Could you check a few things on this model? Use its own coordinates, in mm. Face numbers are marked on the shaded views. A direction names the side the tool comes from. Coordinates: 2 decimals unless noted, no trailing zeros. Loops run counter-clockwise (first coordinate to the right, second up) from the corner with the lowest first, then second, coordinate; pieces in that order, holes last.
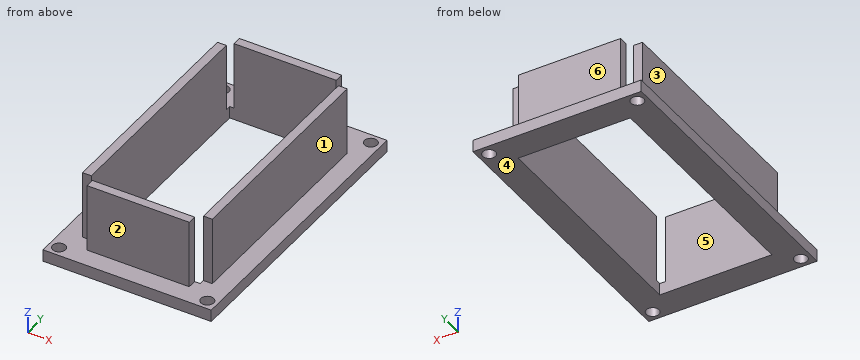
from build123d import *

# Parameters (mm, degrees)
F0_W     = 42
F0_H     = 72
F0_R     = 1.6
F1_DEPTH = 3
F0_W_2   = 25.488504
F0_H_2   = 2.2
F0_W_3   = 2.2
F0_H_3   = 55.283766
F2_DEPTH = 20


with BuildPart() as f1:
    # F0 (on Top) → F1 (new body)
    with BuildSketch(Plane.XY):
        with Locations((-2.088945, 1.718141)):
            Rectangle(F0_W, F0_H)
        with Locations((-20.588945, -31.781859)):
            Circle(F0_R, mode=Mode.SUBTRACT)
        with Locations((16.411055, -31.781859)):
            Circle(F0_R, mode=Mode.SUBTRACT)
        with Locations((-20.588945, 35.218141)):
            Circle(F0_R, mode=Mode.SUBTRACT)
        Polygon((-18.288945, 32.918141), (-14.99591, 32.918141), (10.492594, 32.918141), (14.111055, 32.918141), (14.111055, 29.307075), (14.111055, -25.976691), (14.111055, -27.281859), (14.111055, -29.481859), (10.492594, -29.481859), (-14.99591, -29.481859), (-18.288945, -29.481859), (-18.288945, -25.976691), (-18.288945, 29.307075), align=None, mode=Mode.SUBTRACT)
        with Locations((16.411055, 35.218141)):
            Circle(F0_R, mode=Mode.SUBTRACT)
        Polygon((-16.088945, -27.281859), (-16.088945, -25.976691), (-18.288945, -25.976691), (-18.288945, -29.481859), (-14.99591, -29.481859), (-14.99591, -27.281859), align=None)
        Polygon((-16.088945, 29.307075), (-16.088945, 30.718141), (-14.99591, 30.718141), (-14.99591, 32.918141), (-18.288945, 32.918141), (-18.288945, 29.307075), align=None)
        Polygon((10.492594, 32.918141), (10.492594, 30.718141), (11.911055, 30.718141), (11.911055, 29.307075), (14.111055, 29.307075), (14.111055, 32.918141), align=None)
        Polygon((14.111055, -25.976691), (11.911055, -25.976691), (11.911055, -27.281859), (10.492594, -27.281859), (10.492594, -29.481859), (14.111055, -29.481859), (14.111055, -27.281859), align=None)
    extrude(amount=F1_DEPTH)

    # F0 (on Top) → F2 (join)
    with BuildSketch(Plane.XY):
        with Locations((-2.251658, 31.818141)):
            Rectangle(F0_W_2, F0_H_2)
        with Locations((-17.188945, 1.665192)):
            Rectangle(F0_W_3, F0_H_3)
        with Locations((13.011055, 1.665192)):
            Rectangle(F0_W_3, F0_H_3)
        with Locations((-2.251658, -28.381859)):
            Rectangle(F0_W_2, F0_H_2)
    extrude(amount=F2_DEPTH)


solid = f1.part
(1) We'd pull the mould along Y, two halves only. Please class the marked faces 4, 5 and 6: +Y half, -Y half, draft (parallel to the pull), parting line (faces both ways), or undercut.
Answers:
face 4: draft
face 5: undercut
face 6: +Y half
(2) For pin 1 (1.8 mm diameter, centred on y = -28.5, z = 7.5, fed in from -X); pin 2 (5 mm diameter, centred on y = -10.5, z = 11, fed in from +X); pin 3 (0.7 mm diameter, centred on y = -28.5, z = 8.5, fed in from +X), each with a flat end and sliding along its axis, tell me the tip position at first contact or that it passes through.
Answers:
pin 1: stops at x = -15
pin 2: stops at x = 14.11
pin 3: stops at x = 10.49
(3) Imagine slicing it at A-A, the plane x = 6.5. Write out the boundary of the cut face in (y, z), and give its area (3 significant figures).
Answers:
outline: (-34.28, 0) - (-27.28, 0) - (-27.28, 20) - (-29.48, 20) - (-29.48, 3) - (-34.28, 3) - close; (30.72, 0) - (37.72, 0) - (37.72, 3) - (32.92, 3) - (32.92, 20) - (30.72, 20) - close
area: 117 mm2
(4) Imagine slicing it at B-B, the plane z = 12.75. Write out the boundary of the cut face in (x, y), and give its area (3 significant figures).
Answers:
outline: (-18.29, -25.98) - (-16.09, -25.98) - (-16.09, 29.31) - (-18.29, 29.31) - close; (-15, -29.48) - (10.49, -29.48) - (10.49, -27.28) - (-15, -27.28) - close; (-15, 30.72) - (10.49, 30.72) - (10.49, 32.92) - (-15, 32.92) - close; (11.91, -25.98) - (14.11, -25.98) - (14.11, 29.31) - (11.91, 29.31) - close
area: 355 mm2
(5) Which directions (+Z, -Z, +X, -X, +Y, -Y) give clear straight access to the entire face, cutting with the end or side of a thin tool? Please do the marked faces 1, 2 and 3.
Answers:
face 1: +Z, +X, +Y, -Y
face 2: +Z, +X, -X, -Y
face 3: +Z, -X, +Y, -Y
(6) Imagine slicing it at C-C, the plane y = -11. Write out the boundary of the cut face in (x, z), and give its area (3 significant figures).
Answers:
outline: (-23.09, 0) - (-16.09, 0) - (-16.09, 20) - (-18.29, 20) - (-18.29, 3) - (-23.09, 3) - close; (11.91, 0) - (18.91, 0) - (18.91, 3) - (14.11, 3) - (14.11, 20) - (11.91, 20) - close
area: 117 mm2
(7) I need wall thicknesses on probe 1 along Y at (x, z) = (5.5, 4); probe 2 along X at (y, z) = (-25, 19); probe 3 along X at (y, z) = (30.5, 2). Which ranges of each line are inside material? Lowest first, please.
Answers:
probe 1: y = -29.48 to -27.28, 30.72 to 32.92
probe 2: x = -18.29 to -16.09, 11.91 to 14.11
probe 3: x = -23.09 to -16.09, 11.91 to 18.91
